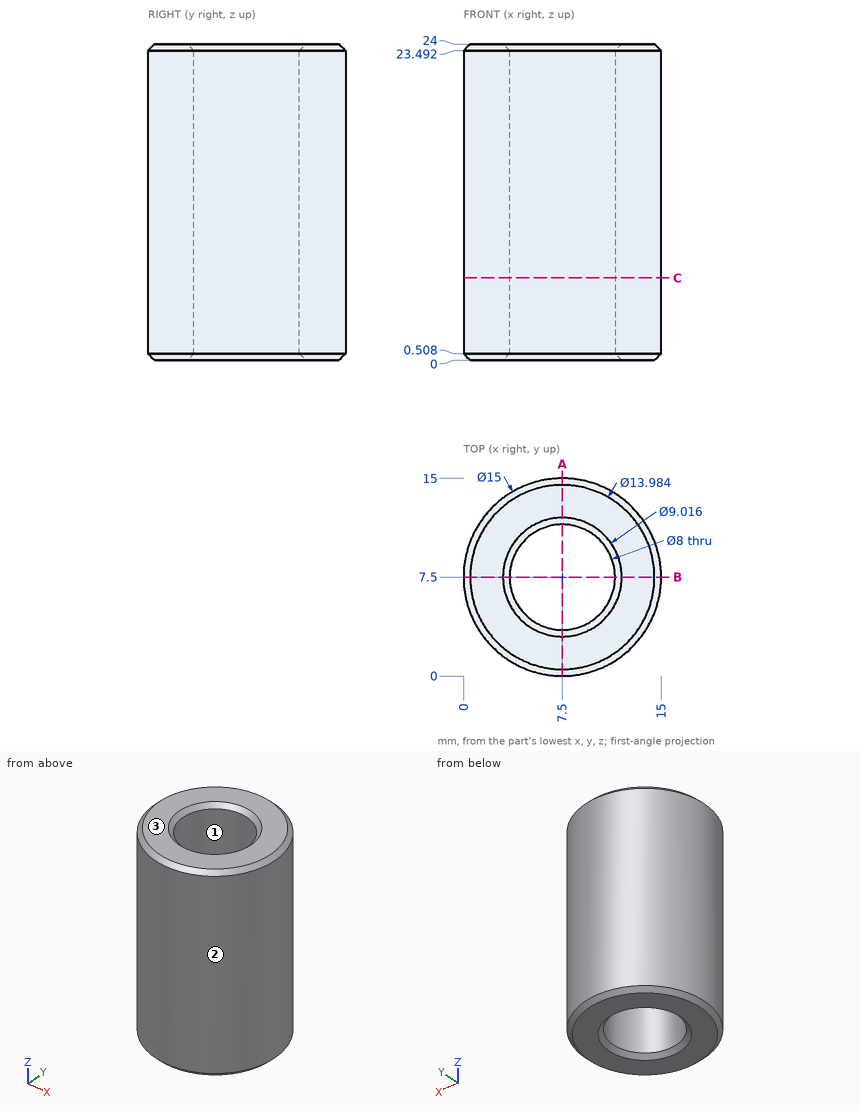
Geometry: see drawing. Coordinates: mm, zero at the bounding-box minimum. Round coordinates to 2 decimals unless told otherwise and drop trailing zeros. Write each loop counter-clockwise with the first axis right and the second up, starting at its lowest first coordinate (ties: lowest second). Pieces come first, ordered by that corner, then holes. Notation, with made-up numbers: M -35.75,-3 L -7.75,-3 A13 ccw -7.75,8 Z; hole C 18,-1.75 d10. An arc over 180 degrees is marked long. Answer as a JSON object with one key per item and string values. Group by question number.
(1) First-contact query: pin 1 (6 mm diameter, centred on y = 2, z = 17, fed in from +X); pin 2 (6 mm diameter, centred on y = 3.5, z = 19.5, fed in from +X); pin 3 (1 mm diameter, centred on y = 4.5, z = 16, fed in from -X). Flat tips, straight axial feed; report the tip coordinate or a pass-through.
(2) Section query A-A on x = 7.5. Output: boundary loops of the cut face in (y, z), then the cut area to 3 significant figures.
(3) Mould query, pull axis X, two halves, no side actions, for the marked faces 1, 2 and 3. Classes: +X half, -X half, draft (parallel to the pull), parting line (faces both ways), or undercut.
(4) Ray query, line 1 (Y direction, x = 7.5, z = 18.75); line 2 (X direction, y = 9.25, z = 7.25); line 3 (X direction, y = 10.75, z = 13.5). Return the intervals inside material, ascending. Write a range as [from, to].
(5) Section query C-C on z = 6.25. Output: boundary loops of the cut face in (x, y), then the cut area to 3 significant figures.
Computed values:
{
 "1": {"pin 1": "x = 14.57", "pin 2": "x = 14.93", "pin 3": "x = 0.43"},
 "2": {"outline": "M 0,0.51 L 0.51,0 L 2.99,0 L 3.5,0.51 L 3.5,23.49 L 2.99,24 L 0.51,24 L 0,23.49 Z; M 11.5,0.51 L 12.01,0 L 14.49,0 L 15,0.51 L 15,23.49 L 14.49,24 L 12.01,24 L 11.5,23.49 Z", "area": "167 mm^2"},
 "3": {"face 1": "undercut", "face 2": "parting line", "face 3": "draft"},
 "4": {"line 1": "[0, 3.5], [11.5, 15]", "line 2": "[0.21, 3.9], [11.1, 14.79]", "line 3": "[0.74, 5.17], [9.83, 14.26]"},
 "5": {"outline": "C 7.5,7.5 d15; hole C 7.5,7.5 d8", "area": "126 mm^2"}
}
